Read the model definition and answer for the solid it produces. Units are mm, in the model's axes. A direction names the side the tool comes from. Round coordinates to 2 decimals unless told otherwise and drop trailing zeros. Order: outer loops, then holes, each group sorted by start corner. A loop starts at its lowest first (then second) coordinate and runs counter-clockwise, first axis right, second up. Notation, with made-up numbers: M -23.75,-21.75 L 13.25,-21.75 A15 ccw 13.25,-5.75 Z; hole C 16,-34.5 d1. An arc over 180 degrees is marked long. Use one line per item in the form item = value. Start each with the question number.
from build123d import *

# Parameters (mm, degrees)
BOSS_EXTRUDE1_DEPTH            = 10
SKETCH5_R                      = 6.75
CUT_EXTRUDE1_DEPTH             = 7
CUT_EXTRUDE1_DIRECTION_2_REACH = 26.463
CUT_EXTRUDE2_REACH             = 8.708
SKETCH6_R                      = 2.5
FILLET1_R                      = 2.5


with BuildPart() as part:
    # Sketch4 → Boss-Extrude1 (new body, symmetric)
    with BuildSketch(Plane(origin=(0, 0, 0), x_dir=(0, 0, -1), z_dir=(1, 0, 0))):
        Polygon((0, 0), (0, 40), (-13.707990749, 40), (-15, 5.56634393), (-32.987342463, 6.241259565), (-32.612389332, 16.2342276), (-37.60887335, 16.421704166), (-38.171303046, 1.432252113), align=None)
    extrude(amount=BOSS_EXTRUDE1_DEPTH, both=True)

    # Sketch5 → Cut-Extrude1 (cut)
    with BuildSketch(Plane.XY.offset(13.707990749)):
        with Locations((0, 28.210852083)):
            Circle(SKETCH5_R)
    extrude(amount=-CUT_EXTRUDE1_DEPTH, mode=Mode.SUBTRACT)

    # Sketch5 → Cut-Extrude1 direction 2 (cut, up to next)
    with BuildSketch(Plane.XY.offset(13.707990749), mode=Mode.PRIVATE) as cut_extrude1_direction_2_sk1:
        with Locations((0, 28.210852083)):
            Circle(SKETCH5_R)
    cut_extrude1_direction_2_tool1 = extrude(cut_extrude1_direction_2_sk1.sketch, amount=CUT_EXTRUDE1_DIRECTION_2_REACH, mode=Mode.PRIVATE) & part.part
    add(cut_extrude1_direction_2_tool1.solids().sort_by_distance((0, 28.210852, 13.707991))[0], mode=Mode.SUBTRACT)

    # Sketch6 → Cut-Extrude2 (cut, up to next)
    with BuildSketch(Plane.XY.offset(6.707990749), mode=Mode.PRIVATE) as cut_extrude2_sk1:
        with Locations((0, 28.210852083)):
            Circle(SKETCH6_R)
    cut_extrude2_tool1 = extrude(cut_extrude2_sk1.sketch, amount=-CUT_EXTRUDE2_REACH, mode=Mode.PRIVATE) & part.part
    add(cut_extrude2_tool1.solids().sort_by_distance((0, 28.210852, 6.707991))[0], mode=Mode.SUBTRACT)

    # Fillet1
    fillet1_edges = [part.edges().sort_by_distance(p)[0] for p in [
        (0, 1.432252113, 38.171303046),
        (0, 16.2342276, 32.612389332),
        (0, 40, 13.707990749),
    ]]
    fillet(fillet1_edges, radius=FILLET1_R)


solid = part.part
Item 1: Section D-D (y = 22) is taken. Write down the section's boundary in (x, z).
Item 2: Section B-B (x = 0) is taken. Write down the section's boundary in (y, z).
Item 3: Find the intervals of material crossed by L1, parallel to Y at x = 0, z = 3.5; L2, parallel to Z at x = 4.75, y = 31.5; L3, parallel to X at y = 28.5, z = 2, in increasing order. Write a range as [from, to].
Item 4: Section A-A (y = 15) is taken. Write down the section's boundary in (x, z), and give its area (3 significant figures).
Item 5: A tool of negligible diameter and unlimited length cuts with its end or side. For faces 1 (the flat face through (0.14, 18.246, 14.524)), 2 (the flat face through (0, 40, 6)), 3 (the flat face through (0.14, 9.94, 32.85)), from which of +Z, -Z, +X, -X, +Y, -Y can it reach the whole face along a straight path? Write none if from no direction.
Item 6: Given P1, Ø6, axis at x = 1, z = 32, coming from the +Y side; P2, Ø4, axis at x = -1, y = 27, coming from the +Z side; P3, Ø4, axis at y = 30.5, z = 18, coming from the -X side; P4, Ø3, axis at x = 1, y = 21.5, coming from the +Z side, each flat-ended and moving along its own axis, determine where each tip first touches the part or whether it passes through.
Item 7: Section C-C (x = -3) is taken. Write down the section's boundary in (y, z), and give its area (3 significant figures).
Item 8: For a pull along Y with two mould halves and no side action, classify faces 4 (the flat face through (0, 25, 6.708)), 5 (the flat face through (0.14, 16.374, 36.342)), 6 (the flat face through (0.14, 0.68, 18.09)), 7 (the cylindrical face through (-1.46, 21.62, 10.53)) as pulls with the +Y half, pulls with the -Y half, needs draft (parallel to the pull), parting line crosses it, or undercut.
The answers:
q1.outline = M -10,0 L 10,0 L 10,14.38 L 2.64,14.38 L 2.64,6.71 L -2.64,6.71 L -2.64,14.38 L -10,14.38 Z
q2.outline = M 0,0 L 25.71,0 L 25.71,6.71 L 21.46,6.71 L 21.46,14.4 L 5.57,15 L 6.24,32.99 L 13.74,32.71 A2.5 ccw 16.33,35.11 L 16.42,37.61 L 3.93,38.08 A2.5 ccw 1.34,35.67 Z; M 30.71,0 L 40,0 L 40,11.3 A2.5 ccw 37.59,13.8 L 34.96,13.9 L 34.96,6.71 L 30.71,6.71 Z
q3.L1 = [0.13, 25.71], [30.71, 40]
q3.L2 = [0, 6.71]
q3.L3 = [-10, -2.48], [2.48, 10]
q4.outline = M -10,0 L 10,0 L 10,14.65 L -10,14.65 Z; M -10,33 L 10,33 L 10,37.66 L -10,37.66 Z
q4.area = 386 mm²
q5.face_1 = +X, -X, +Y
q5.face_2 = +Z, -Z, +X, -X, +Y
q5.face_3 = +X, -X
q6.P1 = 16.32
q6.P2 = 6.71
q6.P3 = through
q6.P4 = 14.46
q7.outline = M 0,0 L 40,0 L 40,11.3 A2.5 ccw 37.59,13.8 L 34.26,13.92 L 34.26,6.71 L 22.16,6.71 L 22.16,14.38 L 5.57,15 L 6.24,32.99 L 13.74,32.71 A2.5 ccw 16.33,35.11 L 16.42,37.61 L 3.93,38.08 A2.5 ccw 1.34,35.67 Z
q7.area = 645 mm²
q8.face_4 = undercut
q8.face_5 = pulls with the +Y half
q8.face_6 = pulls with the -Y half
q8.face_7 = undercut
